from build123d import *

# Parameters (mm, degrees)
SKETCH_1_R                   = 12.5
SKETCH_1_R_2                 = 1.5
EXTRUDE_1_DEPTH              = 10
EXTRUDE_START                = -2
SKETCH_3_R                   = 13.75
SKETCH_3_R_2                 = 12.5
EXTRUDE_3_DEPTH              = 2
SKETCH_4_R                   = 3
CUT_EXTRUDE_1_DEPTH          = 22.866069606
HOLE_WIZARD_M3_1_D           = 4
HOLE_WIZARD_M3_1_CBORE_D     = 7
HOLE_WIZARD_M3_1_CBORE_DEPTH = 8
CHAMFER_1_SIZE               = 0.5
CHAMFER_2_SIZE               = 0.25


with BuildPart() as part:
    # ｽｹｯﾁ1 → ﾎﾞｽ - 押し出し1 (new body)
    with BuildSketch(Plane.XY):
        Circle(SKETCH_1_R)
        with Locations((0, 7.5)):
            Circle(SKETCH_1_R_2, mode=Mode.SUBTRACT)
        with Locations((7.132923872, 2.317627458)):
            Circle(SKETCH_1_R_2, mode=Mode.SUBTRACT)
        with Locations((4.408389392, -6.067627458)):
            Circle(SKETCH_1_R_2, mode=Mode.SUBTRACT)
        with Locations((-4.408389392, -6.067627458)):
            Circle(SKETCH_1_R_2, mode=Mode.SUBTRACT)
        with Locations((-7.132923872, 2.317627458)):
            Circle(SKETCH_1_R_2, mode=Mode.SUBTRACT)
    extrude(amount=EXTRUDE_1_DEPTH)

    # ｽｹｯﾁ3 → ﾎﾞｽ - 押し出し3 (add)
    with BuildSketch(Plane.XY.offset(10).offset(EXTRUDE_START)):
        Circle(SKETCH_3_R)
        Circle(SKETCH_3_R_2, mode=Mode.SUBTRACT)
    extrude(amount=EXTRUDE_3_DEPTH)

    # ｽｹｯﾁ4 → ｶｯﾄ - 押し出し1 (cut, through all)
    with BuildSketch(Plane(origin=(0, 0, 0), x_dir=(-1, 0, 0), z_dir=(0, 0, -1))):
        Circle(SKETCH_4_R)
    extrude(amount=-CUT_EXTRUDE_1_DEPTH, mode=Mode.SUBTRACT)

    # M3 穴付きねじ用座ぐり穴1 (through all)
    with Locations(Plane(origin=(0, 0, 0), x_dir=(-1, 0, 0), z_dir=(0, 0, -1))):
        with Locations((0, 7.5), (7.132923872, 2.317627458), (4.408389392, -6.067627458), (-4.408389392, -6.067627458), (-7.132923872, 2.317627458)):
            CounterBoreHole(HOLE_WIZARD_M3_1_D / 2, HOLE_WIZARD_M3_1_CBORE_D / 2, HOLE_WIZARD_M3_1_CBORE_DEPTH)

    # 面取り1
    chamfer_1_edges = [part.edges().sort_by_distance(p)[0] for p in [
        (-12.5, 0, 0),
        (-13.75, 0, 8),
    ]]
    chamfer(chamfer_1_edges, length=CHAMFER_1_SIZE)

    # 面取り2
    chamfer_2_edges = [part.edges().sort_by_distance(p)[0] for p in [
        (3, 0, 10),
        (3, 0, 0),
        (10.632923872, 2.317627458, 0),
        (7.908389392, -6.067627458, 0),
        (-0.908389392, -6.067627458, 0),
        (-3.632923872, 2.317627458, 0),
        (3.5, 7.5, 0),
    ]]
    chamfer(chamfer_2_edges, length=CHAMFER_2_SIZE)


solid = part.part
Verification items for the finished model (mm, model axes). A direction names the side the tool comes from. Round coordinates to 2 decimals unless told otherwise and drop trailing zeros. Order: outer loops, then holes, each group sorted by start corner. A loop starts at its lowest first (then second) coordinate and runs counter-clockwise, first axis right, second up.
1. Release check for a two-part mould opening along Y. For faces 3 (the cylindrical face through (0.759, 4.083, 4.071)), 4 (the flat face through (3, -3, 10)), 5 (the cylindrical face through (-2.981, -13.423, 9.24)) record: +Y half, -Y half, draft (parallel to the pull), parting line (faces both ways), or undercut.
Final values:
face 3: undercut
face 4: draft
face 5: parting line
2. Section check A-A on x = 0. State how many separate pieces and enclosed holes the cut face has, then the cut area to 3 significant figures.
Final values:
separate pieces: 3
enclosed holes: 0
area: 130 mm2
3. Access from +Z, -Z, +X, -X, +Y, -Y to the whole of each face (thin tool, end or side, straight path). Record for faces 1 (the flat face through (10, 8, 8)), 2 (the cylindrical face through (9, 1.6, 9)).
Final values:
face 1: -Z
face 2: +Z, -Z
4. Thickness scan on L1, parallel to Y at x = 0, z = 6.5; L2, parallel to Y at x = 0, z = 8.6; L3, parallel to X at y = -3.75, z = 2. Record the ranges inside material, lowest first.
Final values:
L1: y = -12.5 to -3, 3 to 4, 11 to 12.5
L2: y = -13.75 to -3, 3 to 5.5, 9.5 to 13.75
L3: x = -11.92 to -7.03, -1.79 to 1.79, 7.03 to 11.92
5. Go/stop test with flat-tipped pins: P1, Ø2, axis at x = -1, y = 6, coming from the -Z side; P2, Ø3.5, axis at x = 7.13, y = 2.32, coming from the +Z side; P3, Ø5, axis at y = -5.5, z = 1.5, coming from the -X side; P4, Ø5, axis at y = 10.5, z = 3, coming from the +X side. Record where each tip stops, or that it passes through.
Final values:
P1: stops at z = 8
P2: passes through
P3: stops at x = -12.13
P4: stops at x = 9.6
6. Section check B-B on z = 2.25. Record the cut outline in (x, y).
Final values:
outline: circle Ø25 at (0, 0); hole circle Ø7 at (-7.13, 2.32); hole circle Ø7 at (-4.41, -6.07); hole circle Ø7 at (0, 7.5); hole circle Ø6 at (0, 0); hole circle Ø7 at (4.41, -6.07); hole circle Ø7 at (7.13, 2.32)
